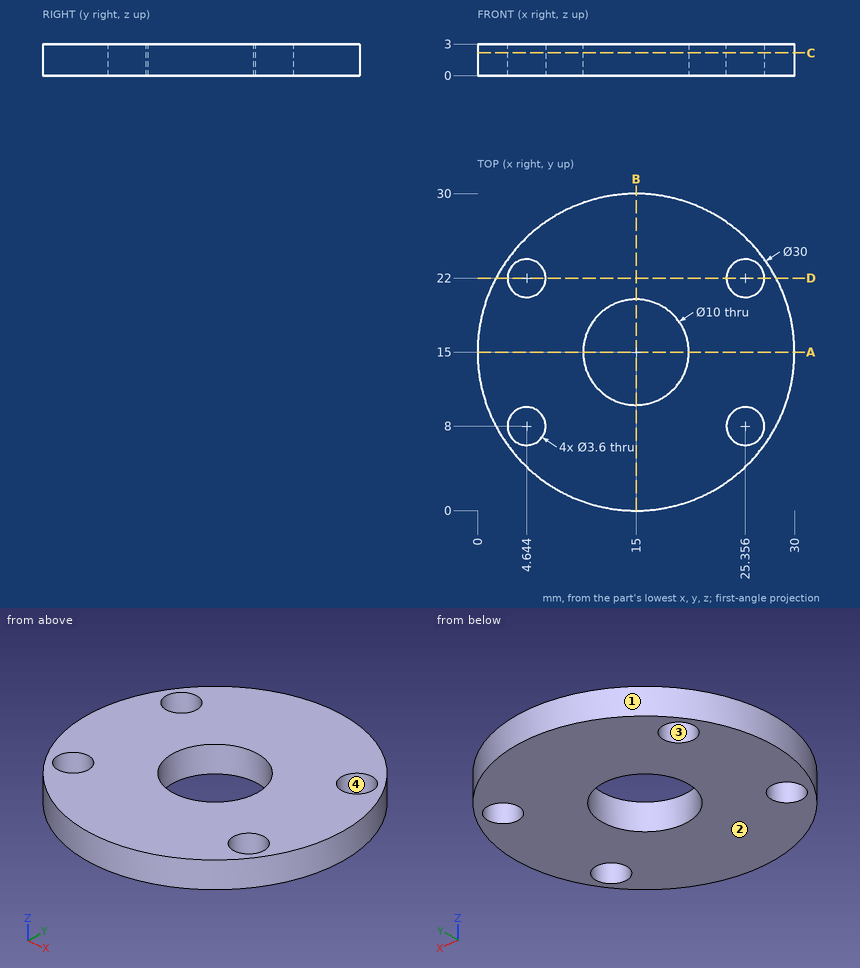
Answer from the drawing. Dimensions are ordinates in mm from the lowest x, y and z of the part. Give positions to 0.01 mm unless a question says otherwise; leave off trailing zeros. Order: outer loops, then holes, each group sorted by start corner. A loop starts at its lowest first (then second) coordinate and runs counter-clockwise, first axis right, second up. Notation, with made-up numbers: (73, -12) - (114, -12) arc R20 cw to (114, -7) - close; hole circle Ø2 at (-12, -9). An arc over 180 degrees is marked (long way). One line per item, written item: value. Start each with the question number.
1) Find the intervals of material crossed by L1, parallel to Y at x = 5.75, z = 2.4; L2, parallel to Y at x = 4.75, z = 0.2; L3, parallel to X at y = 15.25, z = 0.95, in increasing order.
2) The mould has two halves that part along Y. Classify the marked faces 1, 2, 3 and 4: released by +Y, released by -Y, zero draft, split by the parting line, or undercut.
3) Given pin 1 Ø1 at (y, z) = (16.5, 2) entering from -X; pin 2 Ø1.5 at (x, y) = (18.5, 15.5) entering from -Z, each flat-ended and moving along its own axis, determine where each tip first touches the part or whether it passes through.
4) A cutting plane is placed at A-A on y = 15. Give the vertices of the cut face in (x, z), then the cut area to 3 significant figures.
5) A cutting plane is placed at C-C on z = 2.15. Give the vertices of the cut face in (x, y), then the cut area to 3 significant figures.
6) A cutting plane is placed at D-D on y = 22. Give the vertices of the cut face in (x, z).
Answer sheet:
1. L1: y = 3.19 to 6.58, 9.42 to 20.58, 23.42 to 26.81
1. L2: y = 4.05 to 6.2, 9.8 to 20.2, 23.8 to 25.95
1. L3: x = 0 to 10.01, 19.99 to 30
2. face 1: split by the parting line
2. face 2: zero draft
2. face 3: undercut
2. face 4: undercut
3. pin 1: stops at x = 0.03
3. pin 2: passes through
4. outline: (0, 0) - (10, 0) - (10, 3) - (0, 3) - close; (20, 0) - (30, 0) - (30, 3) - (20, 3) - close
4. area: 60.0 mm2
5. outline: circle Ø30 at (15, 15); hole circle Ø3.6 at (4.64, 8); hole circle Ø3.6 at (4.64, 22); hole circle Ø10 at (15, 15); hole circle Ø3.6 at (25.36, 8); hole circle Ø3.6 at (25.36, 22)
5. area: 588 mm2
6. outline: (1.73, 0) - (2.84, 0) - (2.84, 3) - (1.73, 3) - close; (6.44, 0) - (23.56, 0) - (23.56, 3) - (6.44, 3) - close; (27.16, 0) - (28.27, 0) - (28.27, 3) - (27.16, 3) - close
